Check sheet for the modelled part. Datum: model origin and axes. Units: mm. Face numbers are marked on the shaded views. A direction names the side the tool comes from. Give positions to 0.01 mm unless a question says otherwise; leave off trailing zeros. Write each loop counter-clockwise with the first axis right and the second up, starting at its lowest first coordinate (ties: lowest second). Pieces come first, ordered by that corner, then holes. Notation, with made-up numbers: M 46,28.5 L 93,28.5 A22 cw 93,63.5 Z; hole C 0.5,19 d8. An arc over 180 degrees is marked long. Write item = value, one per line. Start each with the question number.
1) Draft check along Z on the marked faces 1, 2 and 3. Enter one of: pulls with the +Z half, pulls with the -Z half, needs draft (parallel to the pull), parting line crosses it, or undercut.
2) Sectioned sample at B-B, the plane z = 15. Record the cut outline in (x, y), then the cut area to 3 significant figures.
3) Sectioned sample at D-D, the plane x = 5. Record the cut outline in (y, z).
4) Gauge pin test, flat ends, axial feed: pin 1 (13 mm diameter, centred on y = -2.06, z = 9.3, fed in from +X); pin 2 (1.5 mm diameter, centred on x = 18, y = 20.5, fed in from +Z); pin 3 (5 mm diameter, centred on x = 15, z = 23, fed in from -Y); pin 4 (2 mm diameter, centred on y = 2.06, z = -9.3, fed in from +X). Record the tip position at first contact, or that the pin passes through.
5) Scan lines: L1, parallel to Y at x = 24, z = 1; L2, parallel to Y at x = 9, z = 9; L3, parallel to Z at x = 16, y = -7.5. Record each from-to range of solid material in increasing order.
6) Sectioned sample at C-C, the plane y = 17.5. Record the cut outline in (x, z), then the cut area to 3 significant figures.
7) Set-up check for the marked faces 4 and 5: record each of +Z, -Z, +X, -X, +Y, -Y from which the full face is reachable in a straight line by a thin tool's end or side.
8) Sectioned sample at A-A, the plane x = 11.5. Record the cut outline in (y, z), then the cut area to 3 significant figures.
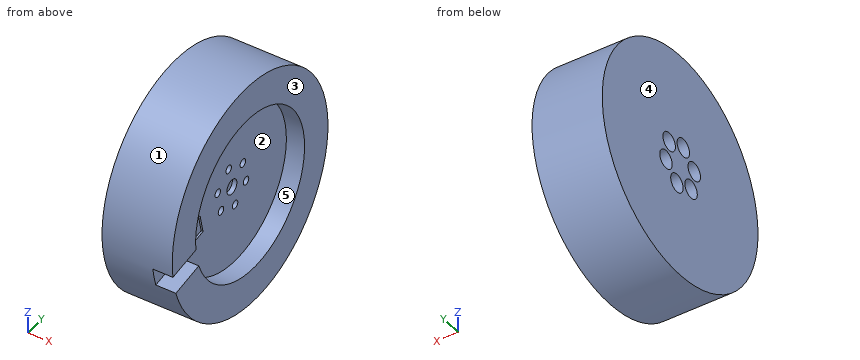
from build123d import *

# Parameters (mm, degrees)
SKETCH1_R           = 50
BOSS_EXTRUDE1_DEPTH = 30.86
SKETCH2_R           = 35
CUT_EXTRUDE1_DEPTH  = 8
CUT_EXTRUDE4_START  = -20
SKETCH10_W          = 10.01875972
SKETCH10_H          = 8.661840267
CUT_EXTRUDE4_DEPTH  = 60
SKETCH12_R          = 3.2
CUT_EXTRUDE5_DEPTH  = 2
SKETCH5_R           = 1.75
CUT_EXTRUDE3_DEPTH  = 30
SKETCH8_R           = 4
CUT_EXTRUDE6_DEPTH  = 10


with BuildPart() as part:
    # Sketch1 → Boss-Extrude1 (new body)
    with BuildSketch(Plane(origin=(0, 0, 0), x_dir=(0, 0, -1), z_dir=(1, 0, 0))):
        Circle(SKETCH1_R)
    extrude(amount=BOSS_EXTRUDE1_DEPTH)

    # Sketch2 → Cut-Extrude1 (cut)
    with BuildSketch(Plane(origin=(30.86, 0, 0), x_dir=(0, 0, -1), z_dir=(1, 0, 0))):
        Circle(SKETCH2_R)
    extrude(amount=-CUT_EXTRUDE1_DEPTH, mode=Mode.SUBTRACT)

    # Sketch10 → Cut-Extrude4 (cut)
    with BuildSketch(Plane(origin=(0, 0, 0), x_dir=(1, 0, 0), z_dir=(0, 0.976356599, 0.21616612)).offset(CUT_EXTRUDE4_START)):
        with Locations((27.048757514, 0.091052199)):
            Rectangle(SKETCH10_W, SKETCH10_H)
    extrude(amount=-CUT_EXTRUDE4_DEPTH, mode=Mode.SUBTRACT)

    # Sketch12 → Cut-Extrude5 (cut)
    with BuildSketch(Plane(origin=(22.86, 0, 0), x_dir=(0, 0, -1), z_dir=(1, 0, 0))):
        Circle(SKETCH12_R)
    extrude(amount=-CUT_EXTRUDE5_DEPTH, mode=Mode.SUBTRACT)

    # Sketch5 → Cut-Extrude3 (cut)
    with BuildSketch(Plane.ZY):
        with Locations((2.868272201, -9.088119419)):
            Circle(SKETCH5_R)
        with Locations((-6.436406189, -7.028056301)):
            Circle(SKETCH5_R)
        with Locations((-9.30467839, 2.060063119)):
            Circle(SKETCH5_R)
        with Locations((-2.868272201, 9.088119419)):
            Circle(SKETCH5_R)
        with Locations((6.436406189, 7.028056301)):
            Circle(SKETCH5_R)
        with Locations((9.30467839, -2.060063119)):
            Circle(SKETCH5_R)
    extrude(amount=-CUT_EXTRUDE3_DEPTH, mode=Mode.SUBTRACT)

    # Sketch8 → Cut-Extrude6 (cut)
    with BuildSketch(Plane.ZY):
        with Locations((-2.868272201, 9.088119419)):
            Circle(SKETCH8_R)
        with Locations((6.436406189, 7.028056301)):
            Circle(SKETCH8_R)
        with Locations((9.30467839, -2.060063119)):
            Circle(SKETCH8_R)
        with Locations((2.868272201, -9.088119419)):
            Circle(SKETCH8_R)
        with Locations((-6.436406189, -7.028056301)):
            Circle(SKETCH8_R)
        with Locations((-9.30467839, 2.060063119)):
            Circle(SKETCH8_R)
    extrude(amount=-CUT_EXTRUDE6_DEPTH, mode=Mode.SUBTRACT)


solid = part.part
Data:
q1.face_1 = parting line crosses it
q1.face_2 = undercut
q1.face_3 = needs draft
q2.outline = M 0,-47.7 L 30.86,-47.7 L 30.86,-31.62 L 22.86,-31.62 L 22.86,31.62 L 30.86,31.62 L 30.86,47.7 L 0,47.7 Z
q2.area = 2,440 mm2
q3.outline = C 0,0 d100; hole C -9.09,2.87 d8; hole C -7.03,-6.44 d8; hole C -2.06,9.3 d8; hole C 2.06,-9.3 d8; hole C 7.03,6.44 d8; hole C 9.09,-2.87 d8
q4.pin_1 = 22.86
q4.pin_2 = 45.93
q4.pin_3 = -45.6
q4.pin_4 = through
q5.L1 = -49.99 to -34.99, 34.99 to 49.99
q5.L2 = -49.18 to -6.05, 1.93 to 3.96, 10.1 to 49.18
q5.L3 = -49.43 to -8.12, -4.75 to 2.13, 3.6 to 49.43
q6.outline = M 0,-46.84 L 30.86,-46.84 L 30.86,-30.31 L 22.86,-30.31 L 22.86,30.31 L 30.86,30.31 L 30.86,46.84 L 0,46.84 Z
q6.area = 2,410 mm2
q7.face_4 = +Z, -Z, -X, +Y, -Y
q7.face_5 = +X
q8.outline = C 0,0 d100; hole C -9.09,2.87 d3.5; hole C -7.03,-6.44 d3.5; hole C -2.06,9.3 d3.5; hole C 2.06,-9.3 d3.5; hole C 7.03,6.44 d3.5; hole C 9.09,-2.87 d3.5
q8.area = 7,800 mm2
